from build123d import *

# Parameters (mm, degrees)
SKETCH1_R           = 7.7
SKETCH1_R_2         = 4.5
BOSS_EXTRUDE1_DEPTH = 12
SKETCH2_R           = 2.15
CUT_EXTRUDE1_DEPTH  = 25
FILLET1_R           = 2


with BuildPart() as part:
    # Sketch1 → Boss-Extrude1 (new body, symmetric)
    with BuildSketch(Plane(origin=(0, 0, 0), x_dir=(0, 0, -1), z_dir=(1, 0, 0))):
        Polygon((15, 10), (15, -15), (-15, -15), (-15, 10), (-15, 40), (15, 40), align=None)
        Circle(SKETCH1_R, mode=Mode.SUBTRACT)
        with Locations((0, 25)):
            Circle(SKETCH1_R_2, mode=Mode.SUBTRACT)
    extrude(amount=BOSS_EXTRUDE1_DEPTH, both=True)

    # Sketch2 → Cut-Extrude1 (cut, through all)
    with BuildSketch(Plane(origin=(12, 0, 0), x_dir=(0, 0, -1), z_dir=(1, 0, 0))):
        with Locations((-9.25, 34.25)):
            Circle(SKETCH2_R)
        with Locations((-9.25, 15.75)):
            Circle(SKETCH2_R)
        with Locations((9.25, 34.25)):
            Circle(SKETCH2_R)
        with Locations((9.25, 15.75)):
            Circle(SKETCH2_R)
    extrude(amount=-CUT_EXTRUDE1_DEPTH, mode=Mode.SUBTRACT)

    # Fillet1
    fillet1_edges = [part.edges().sort_by_distance(p)[0] for p in [
        (0, 40, 15),
        (0, 40, -15),
        (0, -15, -15),
        (0, -15, 15),
    ]]
    fillet(fillet1_edges, radius=FILLET1_R)


solid = part.part
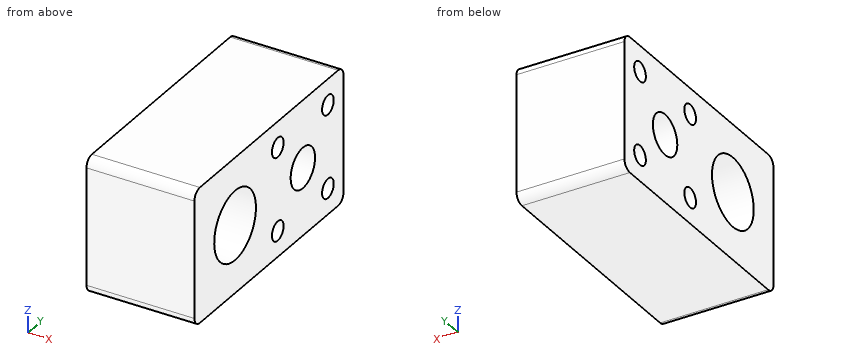
Work out the finished part from the listing and answer in its coordinate system (mm). Give positions to 0.01 mm unless a question says otherwise; leave off trailing zeros. Write each loop counter-clockwise with the first axis right and the second up, starting at its lowest first coordinate (ties: lowest second). Pieces come first, ordered by that corner, then holes.
Q1. The part is cut by section C-C on y = 34.25. Give the vertices of the cut face in (x, z).
Answer:
outline: (-12, -15) - (12, -15) - (12, -11.4) - (-12, -11.4) - close; (-12, -7.1) - (12, -7.1) - (12, 7.1) - (-12, 7.1) - close; (-12, 11.4) - (12, 11.4) - (12, 15) - (-12, 15) - close
Q2. The part is cut by section A-A on x = -10. Give the vertices of the cut face in (y, z), and give its area (3 significant figures).
Answer:
outline: (-15, -13) arc R2 ccw to (-13, -15) - (38, -15) arc R2 ccw to (40, -13) - (40, 13) arc R2 ccw to (38, 15) - (-13, 15) arc R2 ccw to (-15, 13) - close; hole circle Ø15.4 at (0, 0); hole circle Ø4.3 at (15.75, -9.25); hole circle Ø4.3 at (15.75, 9.25); hole circle Ø9 at (25, 0); hole circle Ø4.3 at (34.25, -9.25); hole circle Ø4.3 at (34.25, 9.25)
area: 1,340 mm2
Q3. Straight lines are drawn through the part: L1, parallel to Y at x = -6.75, z = -9.25; L2, parallel to Y at x = 5.75, z = 0; L3, parallel to Z at x = -9.75, y = 34.5. For each, find the intervals that lie inside material, in ascending order.
Answer:
L1: y = -15 to 13.6, 17.9 to 32.1, 36.4 to 40
L2: y = -15 to -7.7, 7.7 to 20.5, 29.5 to 40
L3: z = -15 to -11.39, -7.11 to 7.11, 11.39 to 15
Q4. Given pin 1 (3.5 mm diameter, centred on y = 15.75, z = 9.25, fed in from +X); pin 2 (5.5 mm diameter, centred on y = 34.25, z = 9.25, fed in from +X), each flat-ended and moving along its own axis, determine where each tip first touches the part or whether it passes through.
Answer:
pin 1: passes through
pin 2: stops at x = 12
Q5. The part is cut by section B-B on z = 0. Give the vertices of the cut face in (x, y), and give its area (3 significant figures).
Answer:
outline: (-12, -15) - (12, -15) - (12, -7.7) - (-12, -7.7) - close; (-12, 7.7) - (12, 7.7) - (12, 20.5) - (-12, 20.5) - close; (-12, 29.5) - (12, 29.5) - (12, 40) - (-12, 40) - close
area: 734 mm2
